Can you work these out from the drawing? Everything is in mm from the part's minimum corner. A direction names the side the tool comes from. Round coordinates to 2 decimals unless told otherwise and drop trailing zeros. Write each loop counter-clockwise with the first axis right and the second up, starting at its lowest first coordinate (ties: lowest second). Pieces come first, ordered by that corner, then holes. Notation, with made-up numbers: (33.25, -4.5) -> (56.25, -4.5) arc R30 cw to (56.25, 17.5) -> close; hole circle Ø9 at (78.25, 56). An arc over 180 degrees is marked (long way). Put each result on its own line as item: value. Start each with the question number.
1. We'd pull the mould along Z, two halves only. Please class the marked faces 3, 4, 5 and 6: +Z half, -Z half, draft (parallel to the pull), parting line (faces both ways), or undercut.
2. For pin 1 (1.5 mm diameter, centred on y = 2.5, z = 19.5, fed in from +X); pin 2 (1 mm diameter, centred on y = 2.5, z = 6, fed in from -X); pin 3 (1 mm diameter, centred on x = 4, y = 2.5, fed in from +Z), each with a flat end and sliding along its axis, tell me the tip position at first contact or that it passes through.
3. Which directions (+Z, -Z, +X, -X, +Y, -Y) give clear straight access to the entire face, cutting with the end or side of a thin tool? Please do the marked faces 1 and 2.
4. I need wall thicknesses on probe 1 along Z at (x, y) = (11.25, 0.4) (1 decimal); probe 2 along X at (y, z) = (0.85, 14); probe 3 along Z at (x, y) = (12, 2.95) (1 decimal). Which ranges of each line are inside material? Lowest first, please. Write a range as from..to.
5. Suppose I cut it at C-C (y = 2.5). Please give me the cut outline in (x, z) (1 decimal), then the cut area to 3 significant figures.
6. Suppose I cut it at B-B (x = 12.7). Please give me the cut outline in (y, z) (1 decimal).
7. Suppose I cut it at A-A (z = 12.7). Please give me the cut outline in (x, y) (1 decimal).
8. Suppose I cut it at D-D (x = 19.25). Please give me the cut outline in (y, z) (1 decimal), then the cut area to 3 significant figures.
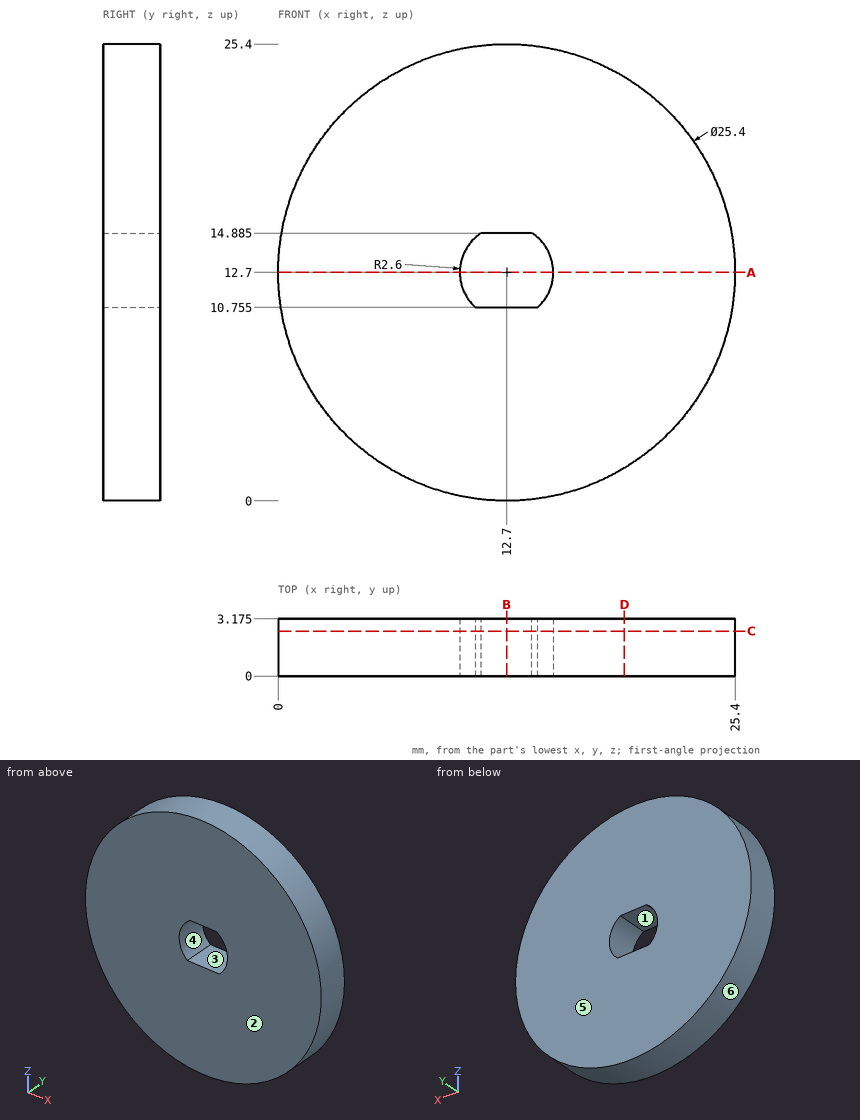
Verdict:
1. face 3: undercut
1. face 4: undercut
1. face 5: draft
1. face 6: parting line
2. pin 1: stops at x = 23.87
2. pin 2: stops at x = 1.62
2. pin 3: stops at z = 22.4
3. face 1: +Y, -Y
3. face 2: +Z, -Z, +X, -X, -Y
4. probe 1: z = 0.1..10.8, 14.9..25.3
4. probe 2: x = 0.07..10.45, 14.95..25.33
4. probe 3: z = 0..10.8, 14.9..25.4
5. outline: circle Ø25.4 at (12.7, 12.7); hole (11, 10.8) -> (14.4, 10.8) arc R2.6 ccw to (14.1, 14.9) -> (11.3, 14.9) arc R2.6 ccw to start
5. area: 488 mm^2
6. outline: (0, 0) -> (3.2, 0) -> (3.2, 10.8) -> (0, 10.8) -> close; (0, 14.9) -> (3.2, 14.9) -> (3.2, 25.4) -> (0, 25.4) -> close
7. outline: (0, 0) -> (10.1, 0) -> (10.1, 3.2) -> (0, 3.2) -> close; (15.3, 0) -> (25.4, 0) -> (25.4, 3.2) -> (15.3, 3.2) -> close
8. outline: (0, 1.8) -> (3.2, 1.8) -> (3.2, 23.6) -> (0, 23.6) -> close
8. area: 69.1 mm^2
